Here's how the part is built. I have some questions about the finished solid (model axes, mm). A direction names the side the tool comes from. Round coordinates to 2 decimals unless told otherwise and drop trailing zeros. Write each loop counter-clockwise with the first axis right and the second up, starting at its lowest first coordinate (ties: lowest second). Pieces come first, ordered by that corner, then holes. Notation, with made-up numbers: (9.25, 57) -> (51.25, 57) arc R14 ccw to (51.25, 79) -> close; hole circle Ø11 at (22.25, 35). An arc over 180 degrees is marked (long way). Answer in a Markdown table with one row per item. Add a question column.
Autodesk Inventor part; units mm, degrees
ref_plane "YZ Plane" through (0, 0, 0) normal (1, 0, 0) x (0, 1, 0)
ref_plane "XZ Plane" through (0, 0, 0) normal (0, 1, 0) x (-1, 0, 0)
ref_plane "XY Plane" through (0, 0, 0) normal (0, 0, 1) x (1, 0, 0)
sketch "Sketch1" plane through (0, 0, 0) normal (0, 1, 0) x (-1, 0, 0)
  line L0 (0, 0) -> (-418.1447, 0)
  line L1 (-418.1447, 0) -> (-418.1447, -76.2)
  line L2 (-418.1447, -76.2) -> (0, -76.2)
  line L3 (0, -76.2) -> (0, 0)
  line L4 (0, -76.2) -> (76.2, -76.2)
  line L5 (76.2, -76.2) -> (76.2, 0)
  line L6 (76.2, 0) -> (0, 0)
  line L7 (0, 0) -> (0, -76.2)
  line L8 (0, 0) -> (76.2, 0)
  line L9 (76.2, 0) -> (76.2, 88.9)
  line L10 (76.2, 88.9) -> (0, 88.9)
  line L11 (0, 88.9) -> (0, 0)
  dimension "d0" = 418.1447
  dimension "d1" = 76.2
  dimension "d4" = 76.2
  dimension "d5" = 76.2
  dimension "d6" = 76.2
  dimension "d7" = 88.9
extrude "Extrusion2" add sketch "Sketch1" along normal blind 127
mirror "Mirror1" about plane through (418.1447, 0, 0) normal (1, 0, 0) of "Extrusion2"
fillet "Fillet1" radius 31.75 8 edges at (-76.2, 127, 6.35) (-76.2, 0, 6.35) (418.1447, 127, -76.2) (418.1447, 0, -76.2) (-76.2, 63.5, -76.2) (912.4895, 63.5, -76.2) (912.4895, 127, 6.35) (912.4895, 0, 6.35)
fillet "Fillet2" radius 31.75 5 edges at (912.4895, 63.5, 88.9) (903.1901, 9.2994, 88.9) (858.5145, 0, 88.9) (858.5145, 127, 88.9) (903.1901, 117.7006, 88.9)
fillet "Fillet3" radius 31.75 5 edges at (-66.9006, 117.7006, 88.9) (-76.2, 63.5, 88.9) (-66.9006, 9.2994, 88.9) (-22.225, 0, 88.9) (-22.225, 127, 88.9)
sketch "Sketch3" plane through (880.7395, 31.75, -76.2) normal (0, 0, -1) x (-1, 0, 0)
  line L0 (314.0818, 85.8231) -> (611.0931, 85.8231) construction
  line L1 (611.0931, 85.8231) -> (611.0931, -17.1741) construction
  line L2 (611.0931, -17.1741) -> (314.0818, -17.1741) construction
  line L3 (314.0818, -17.1741) -> (314.0818, 85.8231) construction
  line L4 (925.1895, 63.5) -> (925.1895, 0)
  line L5 (0, 0) -> (0, 63.5)
  point P0 (880.7395, -31.75)
  dimension "d31" = 314.0964
decal "Decal1"
properties part number "Bumper" material "CFRP"
Item 1: On a 3-axis mill with a long thin cutter (end or side, diameter ignored), from which of +Z, -Z, +X, -X, +Y, -Y can I reach the whole of each face in a straight line? I mean faces 1 (the cylindrical face through (858.2, 117.5, 79.8)), 2 (the flat face through (412, 63, 0)). Say none if no direction works.
Item 2: If we section it at D-D on x = 690: Please give me the cut outline in (y, z), then the cut area to 3 significant figures.
Item 3: If we section it at B-B on x = -13: Please give me the cut outline in (y, z).
Item 4: I need wall thicknesses on line 1 along X through (y, z) = (39, 51.5); line 2 along Z through (x, y) = (84, 86); line 3 along X through (y, z) = (55, 77). Which ranges of each line are inside material? Lowest first, please. Write a range as from..to.
Item 5: For P1, Ø1.5, axis at x = 374, y = 113.5, coming from the -Z side; P2, Ø3, axis at y = 98.5, z = 66, coming from the -X side; P3, Ø1.5, axis at x = 232, y = 90, coming from the +Z side, each with a flat end and sliding along its axis, tell me the tip position at first contact or that it passes through.
Item 6: If we section it at C-C on y = 86: Please give me the cut outline in (x, z), then the cut area to 3 significant figures.
Item 7: If we section it at A-A on z = 15: Please give me the cut outline in (x, y), then the cut area to 3 significant figures.
Item 8: If we mould it in two halves opening along X, with no side actions, what happens to faces 3 (the flat face through (836.289, 63, 44)), 4 (the flat face through (425, 0, -27)), 5 (the cylindrical face through (-66.7, 117.9, 7.1))? For each: pulls with the +X half, pulls with the -X half, needs draft (parallel to the pull), parting line crosses it, or undercut.
Results list:
| question | item | result |
|---|---|---|
| 1 | face 1 | +Z, +X, -X, +Y |
| 1 | face 2 | +Z, +Y, -Y |
| 2 | outline | (0, -44.45) arc R31.75 ccw to (31.75, -76.2) -> (95.25, -76.2) arc R31.75 ccw to (127, -44.45) -> (127, 0) -> (0, 0) -> close |
| 2 | area | 9,240 mm² |
| 3 | outline | (0, -44.45) arc R31.75 ccw to (31.75, -76.2) -> (95.25, -76.2) arc R31.75 ccw to (127, -44.45) -> (127, 57.15) arc R31.75 ccw to (95.25, 88.9) -> (31.75, 88.9) arc R31.75 ccw to (0, 57.15) -> close |
| 4 | line 1 | -76.2..0, 836.29..912.49 |
| 4 | line 2 | -76.2..0 |
| 4 | line 3 | -69.23..0, 836.29..905.52 |
| 5 | P1 | z = -70.94 |
| 5 | P2 | x = -75.19 |
| 5 | P3 | z = 0 |
| 6 | outline | (-76.2, -44.45) arc R31.75 ccw to (-44.45, -76.2) -> (880.74, -76.2) arc R31.75 ccw to (912.49, -44.45) -> (912.49, 57.15) arc R31.75 ccw to (880.74, 88.9) -> (836.29, 88.9) -> (836.29, 0) -> (0, 0) -> (0, 88.9) -> (-44.45, 88.9) arc R31.75 ccw to (-76.2, 57.15) -> close |
| 6 | area | 88,000 mm² |
| 7 | outline | (-76.2, 31.75) arc R31.75 ccw to (-44.45, 0) -> (0, 0) -> (0, 127) -> (-44.45, 127) arc R31.75 ccw to (-76.2, 95.25) -> close; (836.29, 0) -> (880.74, 0) arc R31.75 ccw to (912.49, 31.75) -> (912.49, 95.25) arc R31.75 ccw to (880.74, 127) -> (836.29, 127) -> close |
| 7 | area | 18,500 mm² |
| 8 | face 3 | undercut |
| 8 | face 4 | needs draft |
| 8 | face 5 | pulls with the -X half |
